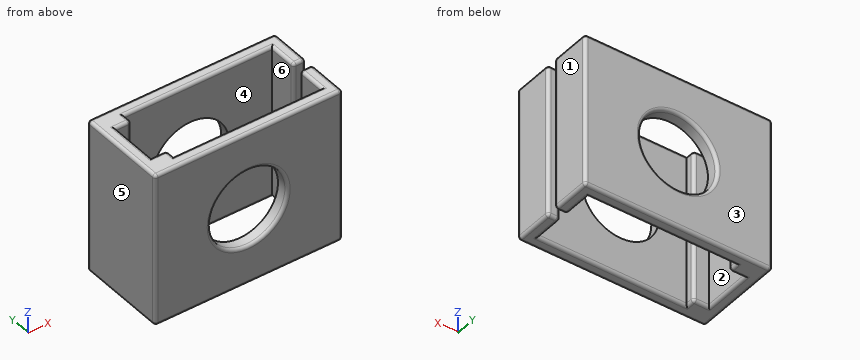
from build123d import *

# Parameters (mm, degrees)
F1_DEPTH = 50
F2_R     = 12.5
F3_DEPTH = 29.501
F6_F1_R  = 1
F6_F2_R  = 1
F6_F3_R  = 1
F6_F4_R  = 1
F6_F5_R  = 1
F6_F6_R  = 1
F6_F7_R  = 1
F6_F8_R  = 1
F6_F9_R  = 1
F6_F10_R = 1
F6_F11_R = 1
F6_F12_R = 1
F6_F13_R = 1
F6_F14_R = 1
F6_F15_R = 1
F6_F16_R = 1
F6_F17_R = 1
F6_F18_R = 1
F6_F19_R = 1
F6_F20_R = 1
F6_F21_R = 1
F6_F22_R = 1
F6_F23_R = 1
F6_F24_R = 1
F6_F25_R = 1


# Not quite as in the source:
# - a feature of the source that left no trace in its solid (it failed there, or was rolled back) is left out


with BuildPart() as f1:
    # F0 (on Top) → F1 (new body)
    with BuildSketch(Plane.XY):
        Polygon((0, 0), (61, 0), (61, 13.25), (57, 13.25), (57, 4), (9, 4), (9, 7), (4, 7), (4, 22.5), (9, 22.5), (9, 25.5), (57, 25.5), (57, 16.25), (61, 16.25), (61, 29.5), (0, 29.5), align=None)
    extrude(amount=F1_DEPTH)

    # F2 (on face) → F3 (cut, through all)
    with BuildSketch(Plane(origin=(0, 29.5, 0), x_dir=(-1, 0, 0), z_dir=(0, 1, 0))):
        with Locations((-30.5, 25)):
            Circle(F2_R)
    extrude(amount=-F3_DEPTH, mode=Mode.SUBTRACT)

    # F6: fillet of radius 1 on 36 edges, made by hand

    # F6_f1
    f6_f1_edges = [f1.edges().sort_by_distance(p)[0] for p in [
        (43, 0, 25),
    ]]
    fillet(f6_f1_edges, radius=F6_F1_R)

    # F6_f2
    f6_f2_edges = [f1.edges().sort_by_distance(p)[0] for p in [
        (43, 29.5, 25),
    ]]
    fillet(f6_f2_edges, radius=F6_F2_R)

    # F6_f3
    f6_f3_edges = [f1.edges().sort_by_distance(p)[0] for p in [
        (30.5, 0, 0),
    ]]
    fillet(f6_f3_edges, radius=F6_F3_R)

    # F6_f4
    f6_f4_edges = [f1.edges().sort_by_distance(p)[0] for p in [
        (30.5, 0, 50),
    ]]
    fillet(f6_f4_edges, radius=F6_F4_R)

    # F6_f5
    f6_f5_edges = [f1.edges().sort_by_distance(p)[0] for p in [
        (30.5, 29.5, 0),
    ]]
    fillet(f6_f5_edges, radius=F6_F5_R)

    # F6_f6
    f6_f6_edges = [f1.edges().sort_by_distance(p)[0] for p in [
        (30.5, 29.5, 50),
    ]]
    fillet(f6_f6_edges, radius=F6_F6_R)

    # F6_f7
    f6_f7_edges = [f1.edges().sort_by_distance(p)[0] for p in [
        (0, 0, 25),
    ]]
    fillet(f6_f7_edges, radius=F6_F7_R)

    # F6_f8
    f6_f8_edges = [f1.edges().sort_by_distance(p)[0] for p in [
        (61, 0, 25),
    ]]
    fillet(f6_f8_edges, radius=F6_F8_R)

    # F6_f9
    f6_f9_edges = [f1.edges().sort_by_distance(p)[0] for p in [
        (61, 13.25, 25),
    ]]
    fillet(f6_f9_edges, radius=F6_F9_R)

    # F6_f10
    f6_f10_edges = [f1.edges().sort_by_distance(p)[0] for p in [
        (61, 29.5, 25),
    ]]
    fillet(f6_f10_edges, radius=F6_F10_R)

    # F6_f11
    f6_f11_edges = [f1.edges().sort_by_distance(p)[0] for p in [
        (57, 13.25, 25),
    ]]
    fillet(f6_f11_edges, radius=F6_F11_R)

    # F6_f12
    f6_f12_edges = [f1.edges().sort_by_distance(p)[0] for p in [
        (9, 7, 25),
    ]]
    fillet(f6_f12_edges, radius=F6_F12_R)

    # F6_f13
    f6_f13_edges = [f1.edges().sort_by_distance(p)[0] for p in [
        (9, 22.5, 25),
    ]]
    fillet(f6_f13_edges, radius=F6_F13_R)

    # F6_f14
    f6_f14_edges = [f1.edges().sort_by_distance(p)[0] for p in [
        (57, 16.25, 25),
    ]]
    fillet(f6_f14_edges, radius=F6_F14_R)

    # F6_f15
    f6_f15_edges = [f1.edges().sort_by_distance(p)[0] for p in [
        (61, 16.25, 25),
    ]]
    fillet(f6_f15_edges, radius=F6_F15_R)

    # F6_f16
    f6_f16_edges = [f1.edges().sort_by_distance(p)[0] for p in [
        (33, 4, 0),
    ]]
    fillet(f6_f16_edges, radius=F6_F16_R)

    # F6_f17
    f6_f17_edges = [f1.edges().sort_by_distance(p)[0] for p in [
        (33, 25.5, 0),
    ]]
    fillet(f6_f17_edges, radius=F6_F17_R)

    # F6_f18
    f6_f18_edges = [f1.edges().sort_by_distance(p)[0] for p in [
        (33, 4, 50),
    ]]
    fillet(f6_f18_edges, radius=F6_F18_R)

    # F6_f19
    f6_f19_edges = [f1.edges().sort_by_distance(p)[0] for p in [
        (33, 25.5, 50),
    ]]
    fillet(f6_f19_edges, radius=F6_F19_R)

    # F6_f20
    f6_f20_edges = [f1.edges().sort_by_distance(p)[0] for p in [
        (4, 14.75, 0),
    ]]
    fillet(f6_f20_edges, radius=F6_F20_R)

    # F6_f21
    f6_f21_edges = [f1.edges().sort_by_distance(p)[0] for p in [
        (4, 14.75, 50),
    ]]
    fillet(f6_f21_edges, radius=F6_F21_R)

    # F6_f22
    f6_f22_edges = [f1.edges().sort_by_distance(p)[0] for p in [
        (6, 7, 0),
    ]]
    fillet(f6_f22_edges, radius=F6_F22_R)

    # F6_f23
    f6_f23_edges = [f1.edges().sort_by_distance(p)[0] for p in [
        (6, 22.5, 0),
    ]]
    fillet(f6_f23_edges, radius=F6_F23_R)

    # F6_f24
    f6_f24_edges = [f1.edges().sort_by_distance(p)[0] for p in [
        (6, 7, 50),
    ]]
    fillet(f6_f24_edges, radius=F6_F24_R)

    # F6_f25
    f6_f25_edges = [f1.edges().sort_by_distance(p)[0] for p in [
        (6, 22.5, 50),
    ]]
    fillet(f6_f25_edges, radius=F6_F25_R)


solid = f1.part
For this review, take the finished solid that the model builds, in its own axes (mm). Face numbers are marked on the shaded views. A direction names the side the tool comes from. Round coordinates to 2 decimals unless told otherwise and drop trailing zeros. Loops run counter-clockwise (first coordinate to the right, second up) from the corner with the lowest first, then second, coordinate; pieces in that order, holes last. Notation, with made-up numbers: (72.25, -24) - (76.25, -24) arc R12 ccw to (76.25, -11) - close; hole circle Ø9 at (-30.75, 79.25). An arc over 180 degrees is marked (long way). One line per question, with ' | ' between items.
Q1. Tool access review of the marked faces 5 and 6: name each direction out of +Z, -Z, +X, -X, +Y, -Y from which nothing blocks a thin tool from reaching the whole face with its end or side.
Taken from the geometry:
face 5: +Z, -Z, -X, +Y, -Y | face 6: +Z, -Z
Q2. For line 1 along X through (y, z) = (25.25, 43.5); line 2 along Y through (x, z) = (7, 37); line 3 along Z through (x, y) = (30.5, 2.05), list the stretches that pass through material, from the lowest coordinate up. Write a range as [from, to].
Taken from the geometry:
line 1: x = [0, 9], [57, 61] | line 2: y = [0, 7], [22.5, 29.5] | line 3: z = [0, 12.5], [37.5, 50]
Q3. Take a section at C-C (x = 30.5). Give the boundary of the cut face in (y, z).
Taken from the geometry:
outline: (0, 1) arc R1 ccw to (1, 0) - (3, 0) arc R1 ccw to (4, 1) - (4, 12.5) - (1, 12.5) arc R1 ccw to (0, 11.5) - close; (0, 38.5) arc R1 ccw to (1, 37.5) - (4, 37.5) - (4, 49) arc R1 ccw to (3, 50) - (1, 50) arc R1 ccw to (0, 49) - close; (25.5, 1) arc R1 ccw to (26.5, 0) - (28.5, 0) arc R1 ccw to (29.5, 1) - (29.5, 11.5) arc R1 ccw to (28.5, 12.5) - (25.5, 12.5) - close; (25.5, 37.5) - (28.5, 37.5) arc R1 ccw to (29.5, 38.5) - (29.5, 49) arc R1 ccw to (28.5, 50) - (26.5, 50) arc R1 ccw to (25.5, 49) - close
Q4. Take a section at A-A (y = 19.5). Give the boundary of the cut face in (x, z), and give its area (3 significant figures).
Taken from the geometry:
outline: (0, 1) arc R1 ccw to (1, 0) - (3, 0) arc R1 ccw to (4, 1) - (4, 49) arc R1 ccw to (3, 50) - (1, 50) arc R1 ccw to (0, 49) - close; (57, 1) arc R1 ccw to (58, 0) - (60, 0) arc R1 ccw to (61, 1) - (61, 49) arc R1 ccw to (60, 50) - (58, 50) arc R1 ccw to (57, 49) - close | area: 398 mm²
Q5. The part is to be moulded in two halves that separate along X. For the marked faces 1, 2, 3 and 4, say which applies: released by +X, released by -X, zero draft, split by the parting line, or undercut.
Taken from the geometry:
face 1: released by +X | face 2: undercut | face 3: zero draft | face 4: undercut
Q6. Take a section at B-B (x = 7). Give the boundary of the cut face in (y, z).
Taken from the geometry:
outline: (0, 1) arc R1 ccw to (1, 0) - (6, 0) arc R1 ccw to (7, 1) - (7, 49) arc R1 ccw to (6, 50) - (1, 50) arc R1 ccw to (0, 49) - close; (22.5, 1) arc R1 ccw to (23.5, 0) - (28.5, 0) arc R1 ccw to (29.5, 1) - (29.5, 49) arc R1 ccw to (28.5, 50) - (23.5, 50) arc R1 ccw to (22.5, 49) - close
Q7. For pin 1 (4.5 mm diameter, centred on y = 16.5, z = 22, fed in from +X), flat-tipped, find the tip position at first contact; note if it passes through.
Taken from the geometry:
pin 1: stops at x = 61
Q8. Take a section at D-D (z = 41.5). Give the boundary of the cut face in (x, y), and give its area (3 significant figures).
Taken from the geometry:
outline: (0, 1) arc R1 ccw to (1, 0) - (60, 0) arc R1 ccw to (61, 1) - (61, 12.25) arc R1 ccw to (60, 13.25) - (58, 13.25) arc R1 ccw to (57, 12.25) - (57, 4) - (9, 4) - (9, 6) arc R1 ccw to (8, 7) - (4, 7) - (4, 22.5) - (8, 22.5) arc R1 ccw to (9, 23.5) - (9, 25.5) - (57, 25.5) - (57, 17.25) arc R1 ccw to (58, 16.25) - (60, 16.25) arc R1 ccw to (61, 17.25) - (61, 28.5) arc R1 ccw to (60, 29.5) - (1, 29.5) arc R1 ccw to (0, 28.5) - close | area: 676 mm²
